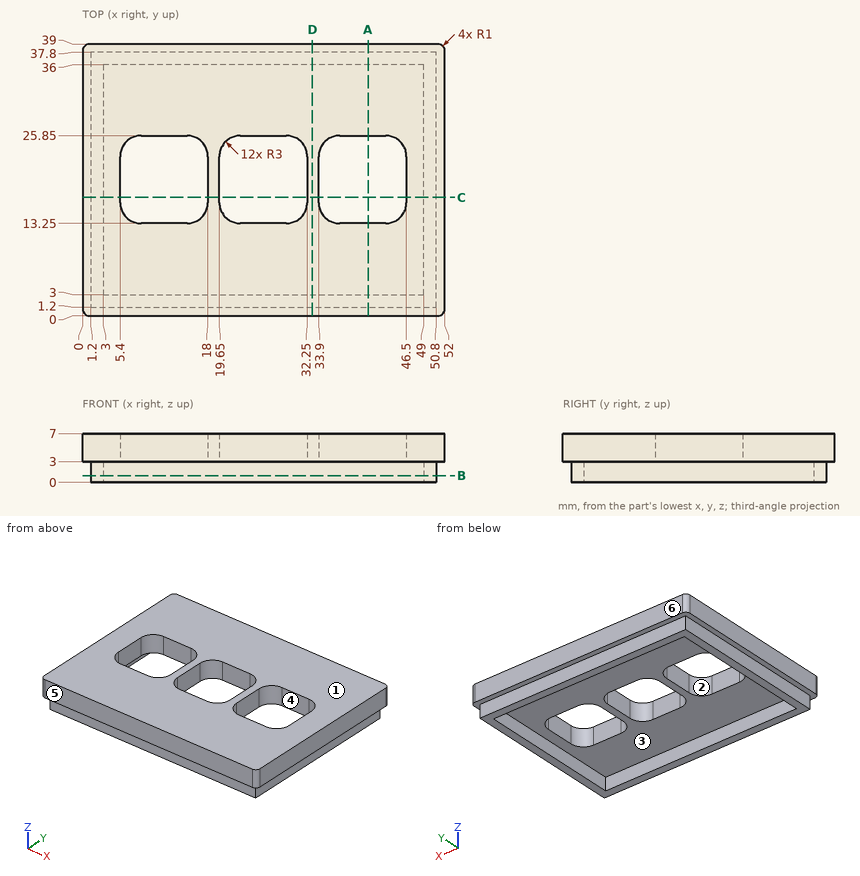
Could you check a few things on this drawing? It's one solid part, dimensions in mm from its lowest x, y, z. A direction names the side the tool comes from. Round coordinates to 2 decimals unless told otherwise and drop trailing zeros. Write each loop counter-clockwise with the first axis right and the second up, starting at its lowest first coordinate (ties: lowest second). Pieces come first, ordered by that corner, then holes.
Q1. Will these pins go through, and if not, where does the flat tip stop? P1, Ø3.5, axis at x = 15, z = 1, coming from the +Y side; P2, Ø10, axis at x = 30, y = 13, coming from the -Z side; P3, Ø1, axis at y = 6.5, z = 1.5, coming from the -X side; P4, Ø4, axis at x = 44, y = 20.5, coming from the -Z side.
Q2. If we mould it in two halves opening along Y, with no side actions, what happens to the marked faces 4, 5 and 6? For each: +Y half, -Y half, draft (parallel to the pull), parting line (faces both ways), or undercut.
Q3. If we section it at C-C on y = 17: Write out the boundary of the cut face in (x, z), plus the area to 3 significant figures.
Q4. If we section it at B-B on z = 1: Write out the boundary of the cut face in (x, y).
Q5. If we section it at D-D on x = 33: Write out the boundary of the cut face in (y, z), plus the area to 3 significant figures.
Q6. Please list where these lines run through material, in increasing order: probe 1 along X at (y, z) = (17, 5.5); probe 2 along Y at (x, z) = (14, 2.25); probe 3 along X at (y, z) = (17.5, 0.75).
Q7. Which directions (+Z, -Z, +X, -X, +Y, -Y) give clear straight access to the entire face, cutting with the end or side of a thin tool? Please do the marked faces 1, 2 and 3.
Q8. If we section it at A-A on x = 41: Write out the boundary of the cut face in (y, z), plus the area to 3 significant figures.
Answer below:
1. P1: stops at y = 37.8
1. P2: stops at z = 3
1. P3: stops at x = 1.2
1. P4: passes through
2. face 4: undercut
2. face 5: -Y half
2. face 6: +Y half
3. outline: (0, 3) - (1.2, 3) - (1.2, 0) - (3, 0) - (3, 3) - (5.4, 3) - (5.4, 7) - (0, 7) - close; (18, 3) - (19.65, 3) - (19.65, 7) - (18, 7) - close; (32.25, 3) - (33.9, 3) - (33.9, 7) - (32.25, 7) - close; (46.5, 3) - (49, 3) - (49, 0) - (50.8, 0) - (50.8, 3) - (52, 3) - (52, 7) - (46.5, 7) - close
3. area: 67.6 mm2
4. outline: (1.2, 1.2) - (50.8, 1.2) - (50.8, 37.8) - (1.2, 37.8) - close; hole (3, 3) - (49, 3) - (49, 36) - (3, 36) - close
5. outline: (0, 3) - (1.2, 3) - (1.2, 0) - (3, 0) - (3, 3) - (36, 3) - (36, 0) - (37.8, 0) - (37.8, 3) - (39, 3) - (39, 7) - (0, 7) - close
5. area: 167 mm2
6. probe 1: x = 0 to 5.4, 18 to 19.65, 32.25 to 33.9, 46.5 to 52
6. probe 2: y = 1.2 to 3, 36 to 37.8
6. probe 3: x = 1.2 to 3, 49 to 50.8
7. face 1: +Z, +X, -X, +Y, -Y
7. face 2: +Z, -Z
7. face 3: -Z
8. outline: (0, 3) - (1.2, 3) - (1.2, 0) - (3, 0) - (3, 3) - (13.25, 3) - (13.25, 7) - (0, 7) - close; (25.85, 3) - (36, 3) - (36, 0) - (37.8, 0) - (37.8, 3) - (39, 3) - (39, 7) - (25.85, 7) - close
8. area: 116 mm2
